For this review, take the finished solid that the model builds, in its own axes (mm). Give positions to 0.01 mm unless a question says otherwise; leave off trailing zeros. Write each loop counter-clockwise with the first axis right and the second up, starting at its lowest first coordinate (ties: lowest second). Pieces come first, ordered by that corner, then holes.
from build123d import *

# Parameters (mm, degrees)
SKETCH1_W           = 95
SKETCH1_H           = 40
SKETCH1_R           = 14
SKETCH1_R_2         = 4.25
BOSS_EXTRUDE1_DEPTH = 6
FILLET1_R           = 10


with BuildPart() as part:
    # Sketch1 → Boss-Extrude1 (new body)
    with BuildSketch(Plane.XY):
        with Locations((347.5, -20)):
            Rectangle(SKETCH1_W, SKETCH1_H)
        with Locations((347.5, -20)):
            Circle(SKETCH1_R, mode=Mode.SUBTRACT)
        with Locations((385, -20)):
            Circle(SKETCH1_R_2, mode=Mode.SUBTRACT)
        with Locations((310, -20)):
            Circle(SKETCH1_R_2, mode=Mode.SUBTRACT)
    extrude(amount=BOSS_EXTRUDE1_DEPTH)

    # Fillet1
    fillet1_edges = [part.edges().sort_by_distance(p)[0] for p in [
        (395, -40, 3),
        (300, -40, 3),
        (300, 0, 3),
        (395, 0, 3),
    ]]
    fillet(fillet1_edges, radius=FILLET1_R)


solid = part.part
(1) We need section D-D (y = -8.5). Write out the cut boundary in (x, z).
(2) We need section C-C (z = 2.1). Write out the cut boundary in (x, y).
(3) Clearance check with flat-ended pins moving along their axes: pin 1 Ø17 at (x, y) = (347.5, -20) entering from +Z; pin 2 Ø1 at (y, z) = (-34.5, 1) entering from +X; pin 3 Ø3 at (y, z) = (-35, 4.5) entering from +X. State where each tip first meets the part, or that it passes through.
(4) The part is to be moulded in two halves that separate along Y. For faces 1 (the flat face through (395, -20, 3)), 2 (the flat face through (347, -40, 3)), 3 (the cylindrical face through (380.754, -19.813, 2.958)), 4 (the cylindrical face through (391.99, -2.85, 3.04)), say which applies: +Y half, -Y half, draft (parallel to the pull), parting line (faces both ways), or undercut.
(5) We need section B-B (y = -20). Write out the cut boundary in (x, z), and give its area (3 significant figures).
(6) We need section A-A (x = 347.5). Write out the cut boundary in (y, z).
(7) For L1, parallel to Y at x = 310, z = 3.6; L2, parallel to X at y = -23.5, z = 0.95; L3, parallel to Y at x = 347.5, z = 2.4, list the stretches that pass through material, from the lowest coordinate up.
The answers:
1. outline: (300.11, 0) - (339.52, 0) - (339.52, 6) - (300.11, 6) - close; (355.48, 0) - (394.89, 0) - (394.89, 6) - (355.48, 6) - close
2. outline: (300, -30) arc R10 ccw to (310, -40) - (385, -40) arc R10 ccw to (395, -30) - (395, -10) arc R10 ccw to (385, 0) - (310, 0) arc R10 ccw to (300, -10) - close; hole circle Ø8.5 at (310, -20); hole circle Ø28 at (347.5, -20); hole circle Ø8.5 at (385, -20)
3. pin 1: passes through
3. pin 2: stops at x = 394.17
3. pin 3: stops at x = 394.37
4. face 1: draft
4. face 2: -Y half
4. face 3: undercut
4. face 4: +Y half
5. outline: (300, 0) - (305.75, 0) - (305.75, 6) - (300, 6) - close; (314.25, 0) - (333.5, 0) - (333.5, 6) - (314.25, 6) - close; (361.5, 0) - (380.75, 0) - (380.75, 6) - (361.5, 6) - close; (389.25, 0) - (395, 0) - (395, 6) - (389.25, 6) - close
5. area: 300 mm2
6. outline: (-40, 0) - (-34, 0) - (-34, 6) - (-40, 6) - close; (-6, 0) - (0, 0) - (0, 6) - (-6, 6) - close
7. L1: y = -40 to -24.25, -15.75 to 0
7. L2: x = 300 to 307.59, 312.41 to 333.94, 361.06 to 382.59, 387.41 to 395
7. L3: y = -40 to -34, -6 to 0
